from build123d import *

# Parameters (mm, degrees)
F0_W     = 70
F0_H     = 280
F1_DEPTH = 24
F2_R     = 7.325
F3_DEPTH = 9
F4_R     = 4.5
F5_DEPTH = 24.001
F7_D     = 6.8


with BuildPart() as f1:
    # F0 (on Top) → F1 (new body)
    with BuildSketch(Plane.XY):
        with Locations((35, 140)):
            Rectangle(F0_W, F0_H)
    extrude(amount=F1_DEPTH)

    # F2 (on face) → F3 (cut)
    with BuildSketch(Plane.XY.offset(24)):
        with Locations((20, 140)):
            Circle(F2_R)
        with Locations((50, 140)):
            Circle(F2_R)
        with Locations((20, 240)):
            Circle(F2_R)
        with Locations((50, 240)):
            Circle(F2_R)
        with Locations((20, 40)):
            Circle(F2_R)
        with Locations((50, 40)):
            Circle(F2_R)
    extrude(amount=-F3_DEPTH, mode=Mode.SUBTRACT)

    # F4 (on face) → F5 (cut, through all)
    with BuildSketch(Plane.XY.offset(24)):
        with Locations((20, 240)):
            Circle(F4_R)
        with Locations((50, 240)):
            Circle(F4_R)
        with Locations((20, 140)):
            Circle(F4_R)
        with Locations((50, 140)):
            Circle(F4_R)
        with Locations((20, 40)):
            Circle(F4_R)
        with Locations((50, 40)):
            Circle(F4_R)
    extrude(amount=-F5_DEPTH, mode=Mode.SUBTRACT)

    # F7 (through all)
    with Locations(Plane.XY.offset(24)):
        with Locations((8.25, 264.75), (61.75, 264.75), (20, 175.5), (50, 175.5), (20, 104.5), (50, 104.5), (8.25, 15.25), (61.75, 15.25)):
            Hole(F7_D / 2)


solid = f1.part
Design review of the part built by this model. Coordinates are the model's own, in mm. A direction names the side the tool comes from. Round coordinates to 2 decimals unless told otherwise and drop trailing zeros. Write each loop counter-clockwise with the first axis right and the second up, starting at its lowest first coordinate (ties: lowest second). Pieces come first, ordered by that corner, then holes. Notation, with made-up numbers: M 57.5,59 L 101.5,59 A30 cw 101.5,81 Z; hole C 30.25,29 d4. An arc over 180 degrees is marked long. One line per item, written item: value. Start each with the question number.
1. To check wall thickness, follow probe 1 along Y at (x, z) = (19.5, 5.25); probe 2 along Y at (x, z) = (50.5, 19.5); probe 3 along Y at (x, z) = (10, 9). State the ranges of each line that lie inside material, in increasing order. Write a range as from..to.
2. Take a section at D-D on y = 140. State the section outline as (x, z) points (3 decimals).
3. Draft analysis for pull direction X (two halves, no side actions). For faces 1 (the face through (49.046, 147.263, 19.563)), 2 (the face through (35, 142, 24)), 3 (the face through (70, 138, 12)), 4 (the face through (16.6, 236.8, 15)), state which applies: pulls with the +X half, pulls with the -X half, needs draft (parallel to the pull), parting line crosses it, or undercut.
4. Take a section at A-A on y = 15.25. State the section outline as (x, z) points.
5. For faces 5 (the face through (14.6, 244.95, 19.56)), 6 (the face through (46.86, 103.2, 11.83)), list the 3-axis set-ups (+Z, -Z, +X, -X, +Y, -Y) from which the entire face can be reached by the end or side of a thin tool; tool diameter is ignored.
6. Take a section at C-C on z = 20.5. State how many separate pieces and enclosed holes the cut face has, then the cut area to 3 significant figures.
7. Take a section at B-B on x = 8.25. State the section outline as (y, z) points.
8. Clearance check with flat-ended pins moving along their axes: P1, Ø9, axis at x = 20, y = 175.5, coming from the +Z side; P2, Ø7.5, axis at x = 17.5, y = 140, coming from the +Z side. State where each tip first meets the part, or that it passes through.
Computed:
1. probe 1: y = 0..35.53, 44.47..101.14, 107.86..135.53, 144.47..172.14, 178.86..235.53, 244.47..280
1. probe 2: y = 0..32.69, 47.31..101.14, 107.86..132.69, 147.31..172.14, 178.86..232.69, 247.31..280
1. probe 3: y = 0..12.33, 18.17..261.83, 267.67..280
2. outline: M 0,0 L 15.5,0 L 15.5,15 L 12.675,15 L 12.675,24 L 0,24 Z; M 24.5,0 L 45.5,0 L 45.5,15 L 42.675,15 L 42.675,24 L 27.325,24 L 27.325,15 L 24.5,15 Z; M 54.5,0 L 70,0 L 70,24 L 57.325,24 L 57.325,15 L 54.5,15 Z
3. face 1: undercut
3. face 2: needs draft
3. face 3: pulls with the +X half
3. face 4: undercut
4. outline: M 0,0 L 4.85,0 L 4.85,24 L 0,24 Z; M 11.65,0 L 58.35,0 L 58.35,24 L 11.65,24 Z; M 65.15,0 L 70,0 L 70,24 L 65.15,24 Z
5. face 5: +Z
5. face 6: +Z, -Z
6. separate pieces: 1
6. enclosed holes: 14
6. area: 18,300 mm²
7. outline: M 0,0 L 11.85,0 L 11.85,24 L 0,24 Z; M 18.65,0 L 261.35,0 L 261.35,24 L 18.65,24 Z; M 268.15,0 L 280,0 L 280,24 L 268.15,24 Z
8. P1: stops at z = 24
8. P2: stops at z = 15
